from build123d import *

# Parameters (mm, degrees)
SKETCH1_W               = 287.02
SKETCH1_H               = 25.4
BOSS_EXTRUDE1_DEPTH     = 3.175
SKETCH2_R               = 3.175
CUT_EXTRUDE1_DEPTH      = 1
CUT_EXTRUDE1_DEPTH_BACK = 7.35


with BuildPart() as part:
    # Sketch1 → Boss-Extrude1 (new body, symmetric)
    with BuildSketch(Plane(origin=(0, 0, 0), x_dir=(1, 0, 0), z_dir=(0, 1, 0))):
        Rectangle(SKETCH1_W, SKETCH1_H)
    extrude(amount=BOSS_EXTRUDE1_DEPTH, both=True)

    # Sketch2 → Cut-Extrude1 (cut, two sides)
    with BuildSketch(Plane(origin=(0, 3.175, 0), x_dir=(1, 0, 0), z_dir=(0, 1, 0))) as cut_extrude1_sk:
        with Locations((-130.81, 0)):
            Circle(SKETCH2_R)
        with Locations((-41.91, 0)):
            Circle(SKETCH2_R)
        with Locations((130.81, 0)):
            Circle(SKETCH2_R)
        with Locations((41.91, 0)):
            Circle(SKETCH2_R)
        with Locations((-92.71, 0)):
            Circle(SKETCH2_R)
        with Locations((-67.31, 0)):
            Circle(SKETCH2_R)
        with Locations((67.31, 0)):
            Circle(SKETCH2_R)
        with Locations((92.71, 0)):
            Circle(SKETCH2_R)
    extrude(amount=CUT_EXTRUDE1_DEPTH, mode=Mode.SUBTRACT)
    extrude(cut_extrude1_sk.sketch, amount=-CUT_EXTRUDE1_DEPTH_BACK, mode=Mode.SUBTRACT)


solid = part.part
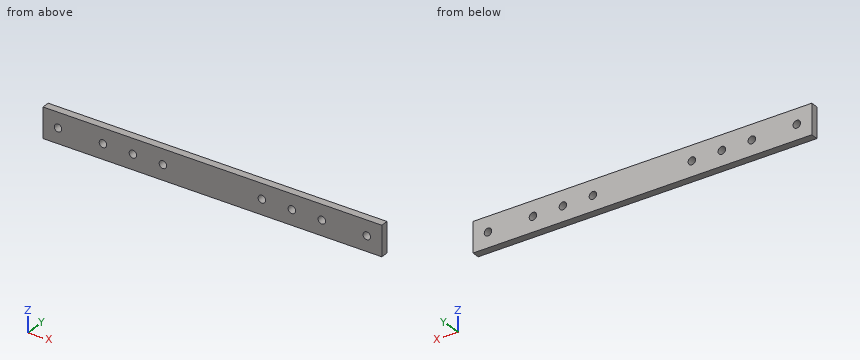
Here's how the part is built. I have some questions about the finished solid (model axes, mm). Give positions to 0.01 mm unless a question says otherwise; leave off trailing zeros. Order: outer loops, then holes, each group sorted by start corner. A loop starts at its lowest first (then second) coordinate and runs counter-clockwise, first axis right, second up. Notation, with made-up numbers: (7, 40) -> (39, 40) arc R13 ccw to (39, 44) -> close; hole circle Ø9 at (87, 30). An arc over 180 degrees is marked (long way). Use a Markdown table: item, result. Add a question column.
Item 1: Imagine slicing it at A-A on y = -2. Give the number of separate pieces and of enclosed holes in the cut face, plus the area to 3 significant figures.
Item 2: Imagine slicing it at B-B on x = -130.81. Please give me the cut outline in (y, z) (3 decimals).
Item 3: I need wall thicknesses on line 1 (Z direction, x = 67.31, y = -0.75) (3 decimals); line 2 (Z direction, x = -131.5, y = 0.75). Which ranges of each line are inside material? Lowest first, please.
Data:
| question | item | result |
|---|---|---|
| 1 | separate pieces | 1 |
| 1 | enclosed holes | 8 |
| 1 | area | 7,040 mm² |
| 2 | outline | (-3.175, -12.7) -> (3.175, -12.7) -> (3.175, -3.175) -> (-3.175, -3.175) -> close; (-3.175, 3.175) -> (3.175, 3.175) -> (3.175, 12.7) -> (-3.175, 12.7) -> close |
| 3 | line 1 | z = -12.7 to -3.175, 3.175 to 12.7 |
| 3 | line 2 | z = -12.7 to -3.1, 3.1 to 12.7 |
